from build123d import *

# Parameters (mm, degrees)
SKETCH_W        = 102.18
SKETCH_H        = 34.92
PAD_DEPTH       = 2
PAD001_DEPTH    = 2
SKETCH002_R     = 15.755262
PAD002_DEPTH    = 4
SKETCH003_R     = 4.859631
PAD003_DEPTH    = 35
SKETCH004_R     = 10
POCKET_DEPTH    = 0.5
SKETCH005_R     = 10
POCKET001_DEPTH = 0.5
SKETCH006_W     = 60
SKETCH006_H     = 20
PAD004_DEPTH    = 10
POCKET002_DEPTH = 3


with BuildPart() as part:
    # Sketch → Pad (new body)
    with BuildSketch(Plane.XY):
        Rectangle(SKETCH_W, SKETCH_H)
    extrude(amount=PAD_DEPTH)

    # Sketch001 → Pad001 (join)
    with BuildSketch(Plane.XY):
        with BuildLine():
            Line((-51.074825, 17.445), (-51.074825, -17.445))
            ThreePointArc((-51.074825, 17.445), (-68.519825, 0), (-51.074825, -17.445))
        make_face()
    extrude(amount=PAD001_DEPTH)

    # Sketch002 (on Face11 of Pad001) → Pad002 (join)
    with BuildSketch(Plane.XY.offset(2)):
        with Locations((-51.87981, 0)):
            Circle(SKETCH002_R)
    extrude(amount=PAD002_DEPTH)

    # Sketch003 (on Face15 of Pad002) → Pad003 (join)
    with BuildSketch(Plane.XY.offset(6)):
        with Locations((-52.405182, 0)):
            Circle(SKETCH003_R)
    extrude(amount=PAD003_DEPTH)

    # Sketch004 (on Face2 of Pad003) → Pocket (cut)
    with BuildSketch(Plane(origin=(0, 0, 0), x_dir=(1, 0, 0), z_dir=(0, 0, -1))):
        with Locations((29.185068, 0)):
            Circle(SKETCH004_R)
    extrude(amount=-POCKET_DEPTH, mode=Mode.SUBTRACT)

    # Sketch005 (on Face2 of Pocket) → Pocket001 (cut)
    with BuildSketch(Plane(origin=(0, 0, 0), x_dir=(1, 0, 0), z_dir=(0, 0, -1))):
        with Locations((-39.903818, 0)):
            Circle(SKETCH005_R)
    extrude(amount=-POCKET001_DEPTH, mode=Mode.SUBTRACT)

    # Sketch006 (on Face4 of Pocket001) → Pad004 (join)
    with BuildSketch(Plane.XY.offset(2)):
        with Locations((10.959466, 0.612018)):
            Rectangle(SKETCH006_W, SKETCH006_H)
    extrude(amount=PAD004_DEPTH)

    # Sketch007 (on DatumPlane) → Pocket002 (cut)
    with BuildSketch(Plane.XY.offset(12)):
        with BuildLine():
            ThreePointArc((-15.157894, 7.560673), (-22.133381, 0.585186), (-15.157894, -6.390301))
            Line((-15.157894, -6.390301), (37.876255, -6.390301))
            ThreePointArc((37.876255, -6.390301), (44.851742, 0.585186), (37.876255, 7.560673))
            Line((37.876255, 7.560673), (-15.157894, 7.560673))
        make_face()
    extrude(amount=-POCKET002_DEPTH, mode=Mode.SUBTRACT)


solid = part.part
CAD build for the part. Positions are in the model's coordinates, mm. A direction names the side the tool comes from. Round coordinates to 2 decimals unless told otherwise and drop trailing zeros. Loops run counter-clockwise (first coordinate to the right, second up) from the corner with the lowest first, then second, coordinate; pieces in that order, holes last.
(1) Which spindle directions (+Z, -Z, +X, -X, +Y, -Y) get a long thin tool onto all of the face, cutting with end or side? Do faces 1 (the cylindrical face through (-57.26, 0.21, 23.26)), 2 (the flat face through (-19.041, 0, 6)), 3 (the flat face through (11, 10.612, 7)). Say none if no direction does.
(2) Cut at D-D (z = 33). Give the cut face in (x, y).
(3) Cut at B-B (z = 4.5). Give the cut face in (x, y).
(4) Two-plate mould, pull along X, no slides. Class faces 4 (the flat face through (-1, 17.46, 1)), 5 (the cylindrical face through (-17.21, -6.08, 10.52)): +X half, -X half, draft (parallel to the pull), parting line (faces both ways), or undercut.
(5) Cut at A-A (x = -5.5). Give the cut face in (y, z).
(6) Drop flat-ended pins along their axis: pin 1 (5 mm diameter, centred on y = -4, z = 33, fed in from -X); pin 2 (8 mm diameter, centred on x = 13.5, z = 8, fed in from -Y); pin 3 (4 mm diameter, centred on x = -36.5, z = 6.5, fed in from +Y). Give the stop position or say it passes through.
(7) Cut at C-C (y = 0). Give the cut face in (x, z), plus the area to 3 significant figures.
(8) Wall check: line 1 along X through (y, z) = (0, 0.3); line 2 along Z through (x, y) = (-27, -15); line 3 along Z through (x, y) = (14, -8). Give the ranges that are in metal, low to high.
Findings below:
1. face 1: +Z
1. face 2: +Z, +Y, -Y
1. face 3: +Z, +X, +Y
2. outline: circle Ø9.72 at (-52.41, 0)
3. outline: circle Ø31.51 at (-51.88, 0); (-19.04, -9.39) - (40.96, -9.39) - (40.96, 10.61) - (-19.04, 10.61) - close
4. face 4: draft
4. face 5: undercut
5. outline: (-17.46, 0) - (17.46, 0) - (17.46, 2) - (10.61, 2) - (10.61, 12) - (7.56, 12) - (7.56, 9) - (-6.39, 9) - (-6.39, 12) - (-9.39, 12) - (-9.39, 2) - (-17.46, 2) - close
6. pin 1: stops at x = -57.03
6. pin 2: stops at y = -9.39
6. pin 3: stops at y = 8.22
7. outline: (-68.52, 0) - (-49.9, 0) - (-49.9, 0.5) - (-29.9, 0.5) - (-29.9, 0) - (19.19, 0) - (19.19, 0.5) - (39.19, 0.5) - (39.19, 0) - (51.09, 0) - (51.09, 2) - (40.96, 2) - (40.96, 9) - (-19.04, 9) - (-19.04, 2) - (-36.12, 2) - (-36.12, 6) - (-47.55, 6) - (-47.55, 41) - (-57.26, 41) - (-57.26, 6) - (-67.64, 6) - (-67.64, 2) - (-68.52, 2) - close
7. area: 1,110 mm2
8. line 1: x = -68.52 to -49.9, -29.9 to 19.19, 39.19 to 51.09
8. line 2: z = 0 to 2
8. line 3: z = 0 to 12
